Geometry: final body of the model. Coordinates: model frame, mm. A direction names the side the tool comes from. Round coordinates to 2 decimals unless told otherwise and drop trailing zeros. Order: outer loops, then holes, each group sorted by start corner. A loop starts at its lowest first (then second) coordinate and runs counter-clockwise, first axis right, second up. Notation, with made-up numbers: (10, 14) - (34, 14) arc R16 cw to (34, 28) - close; hole circle Ø6 at (71, 88.5). An arc over 180 degrees is marked (long way). Put each result on its own line as item: value. Start each with the question number.
(1) Pull-direction query (X, two-part tool) for faces 1 (the face through (-1.5, 0.07, 53.24)), 2 (the face through (0, -2, 105)), 3 (the face through (-1.08, -4.88, 51.33)); classes: released by +X, released by -X, zero draft, split by the parting line, or undercut.
(2) Section A-A (x = 0). Output: boundary loops of the cut face in (y, z), and give its area (3 significant figures).
(3) Pin query (flat end, axial travel): P1, Ø4, axis at y = 3, z = 92.5, coming from the -X side; P2, Ø1, axis at y = -6.5, z = 85.5, coming from the -X side; P3, Ø1.5, axis at y = -2, z = 28, coming from the +X side; P4, Ø1.5, axis at x = 3, y = -6, coming from the +Z side. Return the tip coordinate at first contact, or that it passes through.
(4) Access query for faces 4 (the face through (2, 0, 0)), 5 (the face through (4, -4, 4)). Directions: +Z, -Z, +X, -X, +Y, -Y. A direction counts if a zero-diameter tool reaches every point of the face in a straight line with its end or side. Return the directions, or none.
(5) Section C-C (z = 19). Output: boundary loops of the cut face in (x, y).
(6) Material intervals for L1, parallel to Y at x = 0, z = 65.5; L2, parallel to X at y = -0.5, z = 40.5; L3, parallel to Y at x = -1, z = 40.5, sorted ascending. Write a range as [from, to].
(7) Section D-D (y = -7.5). Output: boundary loops of the cut face in (x, z).
from build123d import *

# Parameters (mm, degrees)
F0_R     = 8.5
F1_DEPTH = 4
F2_R     = 5
F3_DEPTH = 100
F4_W     = 4
F4_H     = 5
F6_R     = 1.5
F7_DEPTH = 112


with BuildPart() as f1:
    # F0 (on Top) → F1 (new body)
    with BuildSketch(Plane.XY):
        Circle(F0_R)
    extrude(amount=F1_DEPTH)

    # F2 (on Top) → F3 (join)
    with BuildSketch(Plane.XY):
        Circle(F2_R)
    extrude(amount=F3_DEPTH)

    # F4 (on Right) → F5 (revolve)
    with BuildSketch(Plane.YZ):
        with Locations((2, 102.5)):
            Rectangle(F4_W, F4_H)
    revolve(axis=Axis((0, 0, 102.5), (0, 0, -1)))

    # F6 (on face) → F7 (cut)
    with BuildSketch(Plane.XY.offset(105)):
        Circle(F6_R)
    extrude(amount=-F7_DEPTH, mode=Mode.SUBTRACT)


solid = f1.part
Checks:
1. face 1: undercut
1. face 2: zero draft
1. face 3: split by the parting line
2. outline: (-8.5, 0) - (-1.5, 0) - (-1.5, 105) - (-4, 105) - (-4, 100) - (-5, 100) - (-5, 4) - (-8.5, 4) - close; (1.5, 0) - (8.5, 0) - (8.5, 4) - (5, 4) - (5, 100) - (4, 100) - (4, 105) - (1.5, 105) - close
2. area: 753 mm²
3. P1: stops at x = -4.9
3. P2: passes through
3. P3: stops at x = 4.84
3. P4: stops at z = 4
4. face 4: -Z, +X, -X, +Y, -Y
4. face 5: +Z
5. outline: circle Ø10 at (0, 0); hole circle Ø3 at (0, 0)
6. L1: y = [-5, -1.5], [1.5, 5]
6. L2: x = [-4.97, -1.41], [1.41, 4.97]
6. L3: y = [-4.9, -1.12], [1.12, 4.9]
7. outline: (-4, 0) - (4, 0) - (4, 4) - (-4, 4) - close
